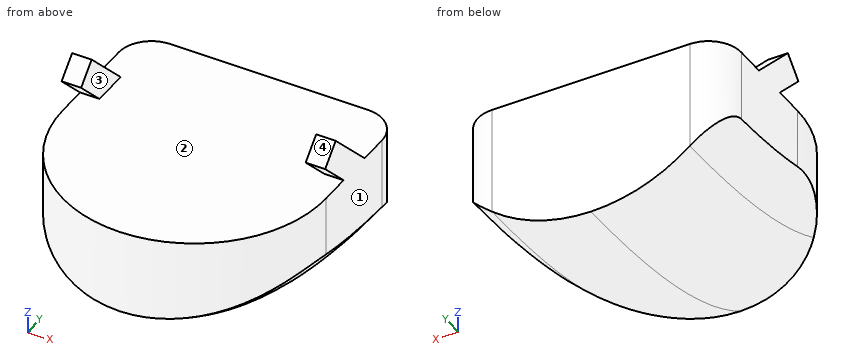
Autodesk Inventor part; units mm, degrees
ref_plane "Dovetail Plane" through (-10, 13.75, 0) normal (0, -0.7071068, 0.7071068) x (1, 0, 0)
ref_plane "MidPlane" through (0, 10, -11) normal (1, 0, 0) x (0, 0, -1)
ref_plane "YZ Plane" through (0, 0, 0) normal (1, 0, 0) x (0, 1, 0)
sketch "Imprint Transfer" plane through (0, 0, 0) normal (0, 0, 1) x (1, 0, 0)
  arc A0 (-10, 10) -> (10, 10) centre (0, 10) ccw
  line L0 (10, 10) -> (10, 17.5)
  arc A1 (10, 17.5) -> (7.5, 20) centre (7.5, 17.5) ccw
  line L1 (7.5, 20) -> (-7.5, 20)
  arc A2 (-7.5, 20) -> (-10, 17.5) centre (-7.5, 17.5) ccw
  line L2 (-10, 17.5) -> (-10, 10)
  point P0 (0, 0)
  point P1 (0, 7.0711)
sketch "Sketch2" plane through (0, 0, 0) normal (0, 0, 1) x (1, 0, 0)
  line L0 (-10, 17.5) -> (-10, 10)
  arc A0 (-10, 10) -> (10, 10) centre (0, 10) ccw
  line L1 (10, 10) -> (10, 17.5)
  arc A1 (10, 17.5) -> (7.5, 20) centre (7.5, 17.5) ccw
  line L2 (7.5, 20) -> (-7.5, 20)
  arc A2 (-7.5, 20) -> (-10, 17.5) centre (-7.5, 17.5) ccw
  point P0 (0, 0)
extrude "Extrusion1" add sketch "Sketch2" against normal blind 11
sketch "Rotational Axis" plane through (0, 0, 0) normal (0, 0, 1) x (1, 0, 0)
  arc A0 (-10, 10) -> (10, 10) centre (0, 10) ccw
  line L0 (10, 10) -> (10, 17.5)
  arc A1 (10, 17.5) -> (7.5, 20) centre (7.5, 17.5) ccw
  line L1 (7.5, 20) -> (-7.5, 20)
  arc A2 (-7.5, 20) -> (-10, 17.5) centre (-7.5, 17.5) ccw
  line L2 (-10, 17.5) -> (-10, 10)
  line L3 (-10, 10) -> (-10, 17.5)
  line L4 (-10, 13.75) -> (10, 13.75)
  line L5 (10, 17.5) -> (10, 10)
  point P0 (0, 0)
ref_plane "Dovetail Plane" through (-10, 13.75, 0) normal (0, -0.7071068, 0.7071068) x (1, 0, 0)
sketch "Sketch4" plane through (-10, 13.75, 0) normal (0, -0.7071068, 0.7071068) x (1, 0, 0)
  ellipse E0 centre (10, -2.6517) end of major axis (0, -2.6517) minor radius 7.0711 (0, -2.6517) -> (20, -2.6517) ccw
  line L0 (20, -2.6517) -> (20, 2.6517)
  ellipse E1 centre (17.5, 2.6517) end of major axis (20, 2.6517) minor radius 1.7678 (20, 2.6517) -> (17.5, 4.4194) ccw
  line L1 (17.5, 4.4194) -> (2.5, 4.4194)
  ellipse E2 centre (2.5, 2.6517) end of major axis (0, 2.6517) minor radius 1.7678 (2.5, 4.4194) -> (0, 2.6517) ccw
  line L2 (0, 2.6517) -> (0, -2.6517)
  line L3 (0, 0) -> (20, 0)
  line L4 (0, 1) -> (20, 1)
  line L5 (0, -1) -> (20, -1)
  line L6 (0, 1) -> (1.48, 1)
  line L7 (1.48, 1) -> (1.48, -1)
  line L8 (1.48, -1) -> (0, -1)
  line L9 (0, -1) -> (0, 1)
  line L10 (20, 1) -> (18.52, 1)
  line L11 (18.52, 1) -> (18.52, -1)
  line L12 (18.52, -1) -> (20, -1)
  line L13 (20, -1) -> (20, 1)
  point P0 (10, -9.7227)
  point P1 (1.48, 1)
  point P2 (0, 1)
  point P3 (0, -1)
  point P4 (1.48, -1)
  point P5 (18.52, 1)
  point P6 (18.52, -1)
  point P7 (20, -1)
  point P8 (20, 1)
  dimension "d3" = 1
  dimension "d4" = 1
  dimension "d5" = 1.48
  dimension "d6" = 2
  dimension "d7" = 1.48
  dimension "d8" = 2
  dimension "d13" = 0
  dimension "d14" = 0
extrude "Extrusion2" add sketch "Sketch4" along normal blind 4.5 and the other way blind 2 contours L2 L3 L7 L5 | L5 L11 L3 L0 | L2 L4 L7 L3 | L3 L11 L4 L0
sketch "Sketch6" plane through (-7.5, 20, 0) normal (0, 1, 0) x (1, 0, 0)
  line L0 (15, 0) -> (0, 0)
  line L1 (15, 0) -> (15, 11)
  line L2 (0, 11) -> (15, 11)
  line L3 (0, 0) -> (0, 11)
  line L4 (17.5, 0) -> (15, 0)
  line L5 (17.5, 0) -> (17.5, 11)
  line L6 (15, 11) -> (17.5, 11)
  line L7 (15, 0) -> (15, 11)
  line L8 (0, 0) -> (-2.5, 0)
  line L9 (0, 0) -> (0, 11)
  line L10 (-2.5, 11) -> (0, 11)
  line L11 (-2.5, 0) -> (-2.5, 11)
  line L12 (17.5, 0) -> (17.5, 11)
  line L13 (-2.5, 0) -> (-2.5, 11)
  arc A0 (17.5, 5.5) -> (-2.5, 5.5) centre (7.5, -0.8409) ccw
  line L14 (17.5, 11) -> (-2.5, 11)
  line L15 (-2.5, 11) -> (-2.5, 16)
  line L16 (-2.5, 16) -> (17.5, 16)
  line L17 (17.5, 16) -> (17.5, 11)
  point P0 (7.5, 0)
  point P1 (7.5, 11)
  point P2 (-2.5, 5.5)
  dimension "d27" = 20
  dimension "d28" = 5
ref_plane "MidPlane" through (0, 10, -11) normal (1, 0, 0) x (0, 0, -1)
sketch "GuideReference" plane through (0, 10, -11) normal (1, 0, 0) x (0, 0, -1)
  line L0 (-11, 0) -> (-11, 0)
  line L1 (-11, 0) -> (0, 0)
  line L2 (0, 0) -> (0, 0)
  line L3 (-11, 0) -> (0, 0)
  line L4 (-11, 10) -> (-11, 7.5)
  line L5 (-11, 10) -> (0, 10)
  line L6 (0, 7.5) -> (0, 10)
  line L7 (-11, 7.5) -> (0, 7.5)
  line L8 (-11, 7.5) -> (-11, 5.1642)
  line L9 (-11, 7.5) -> (0, 7.5)
  line L10 (0, 0) -> (0, 7.5)
  line L11 (-11, 0) -> (0, 0)
  line L12 (-11, 2.3358) -> (-11, 0)
  line L13 (-11, 2.3358) -> (-13.4749, -0.1391)
  line L14 (-14.8891, 1.2751) -> (-13.4749, -0.1391)
  line L15 (-11, 5.1642) -> (-14.8891, 1.2751)
  line L16 (-11.8409, -10) -> (-0.8409, -10) construction
  line L17 (-11.8409, 10) -> (-11.8409, -7.5)
  line L18 (-11.8409, 10) -> (5.6591, 10) construction
  line L19 (-11.8409, -7.5) -> (-18.8409, -7.5)
  line L20 (-18.8409, -7.5) -> (-22.8409, -7.5)
  line L21 (-11.8409, 10) -> (-11.8409, -7.5) construction
  line L22 (-11.8409, -7.5) -> (-18.8409, -7.5) construction
  line L23 (-18.8409, -7.5) -> (-22.8409, -7.5) construction
  spline S0 degree 3 poles (-11.8409, 10) (-11.8409, -7.5) (-18.8409, -7.5) (-22.8409, -7.5) knots 1 1 1 1 2 2 2 2
  point P0 (-11, -10)
  dimension "d24" = 17.5
  dimension "d25" = 90
  dimension "d26" = 7
sketch "Sketch10" plane through (0, 10, -11) normal (1, 0, 0) x (0, 0, -1)
  spline S0 degree 3 poles (-11.8409, 10) (-11.8409, -7.5) (-18.8409, -7.5) (-22.8409, -7.5) knots 1 1 1 1 2 2 2 2
  point P0 (-11, -10)
sweep "Sweep2" cut profiles "Sketch6" path "Sketch10" contours A0 L2 L1 | L1 L6 L5 A0 | A0 L11 L10 L3 | L3 L2 A0 | L2 L10 L15 L16 L17 L6
properties part number "FingerTip Hardtip"
The listing builds one solid part. Answer for the finished solid, in the listing's coordinates (mm). Face numbers are marked on the shaded views. Give positions to 0.01 mm unless a question says otherwise; leave off trailing zeros. Loops run counter-clockwise (first coordinate to the right, second up) from the corner with the lowest first, then second, coordinate; pieces in that order, holes last. Notation, with made-up numbers: (17, 22.25) - (29, 22.25) arc R27 cw to (29, 41.25) - close; hole circle Ø1 at (10.25, 22). An arc over 180 degrees is marked (long way). Return JSON: item names as keys, results as strings. Group by question number.
1. Find section A-A (z = -2.75). Write down the section's boundary in (x, y).
2. Straight lines are drawn through the part: line 1 (Y direction, x = 0.25, z = -6); line 2 (Z direction, x = 0.5, y = 11.25); line 3 (X direction, y = 5, z = -8). For each, find the intervals that lie inside material, in ascending order. Write a range as [from, to].
3. Given pin 1 Ø4 at (x, y) = (7, 17) entering from +Z; pin 2 Ø2 at (x, z) = (-2, -4) entering from -Y; pin 3 Ø1 at (x, y) = (-7, 17) entering from -Z, each flat-ended and moving along its own axis, determine where each tip first touches the part or whether it passes through.
4. Determine the mould class of the marked faces 1, 2, 3 and 4 for opening direction X: pulls with the +X half, pulls with the -X half, needs draft (parallel to the pull), parting line crosses it, or undercut.
Verdict:
{
 "1": {"outline": "(-10, 10) arc R10 ccw to (10, 10) - (10, 17.5) arc R2.5 ccw to (7.5, 20) - (-7.5, 20) arc R2.5 ccw to (-10, 17.5) - close"},
 "2": {"line 1": "y = [0, 20]", "line 2": "z = [-10.38, 0]", "line 3": "x = [-4.32, 4.32]"},
 "3": {"pin 1": "stops at z = 0", "pin 2": "stops at y = 0.05", "pin 3": "stops at z = -8.99"},
 "4": {"face 1": "pulls with the +X half", "face 2": "undercut", "face 3": "undercut", "face 4": "needs draft"}
}
